Autodesk Inventor part; units mm, degrees
ref_plane "YZ Plane" through (0, 0, 0) normal (1, 0, 0) x (0, 1, 0)
ref_plane "XZ Plane" through (0, 0, 0) normal (0, 1, 0) x (-1, 0, 0)
ref_plane "XY Plane" through (0, 0, 0) normal (0, 0, 1) x (1, 0, 0)
sketch "草图1" plane through (0, 0, 0) normal (0, 1, 0) x (-1, 0, 0)
  circle A0 centre (0, 0) radius 1.5
  line L0 (0, 0) -> (-13.1253, 0) construction
  circle A1 centre (-4.1, 0) radius 0.5
  circle A2 centre (-6.2, 0) radius 0.5
  circle A3 centre (-8.3, 0) radius 0.5
  circle A4 centre (-10.4, 0) radius 0.5
  circle A5 centre (-12.5, 0) radius 0.5
  circle A6 centre (-14.6, 0) radius 0.5
  arc A7 (-0.4195, -3.4748) -> (-0.4195, 3.4748) centre (0, 0) ccw
  arc A8 (-14.8098, 1.7374) -> (-14.8098, -1.7374) centre (-14.6, 0) ccw
  line L1 (-0.4195, -3.4748) -> (-14.8098, -1.7374)
  line L2 (-0.4195, 3.4748) -> (-14.8098, 1.7374)
  dimension "d0" = 3
  dimension "d1" = 1
  dimension "d2" = 4.1
  dimension "d5" = 2.1
  dimension "d10" = 7
  dimension "d11" = 3.5
extrude "拉伸1" add sketch "草图1" along normal blind 1.5
sketch "草图2" plane through (0, 1.5, 0) normal (0, 1, 0) x (1, 0, 0)
  circle A0 centre (0, 0) radius 3.5
  line L0 (0.4195, -3.4748) -> (14.8098, -1.7374)
  arc A1 (14.8098, -1.7374) -> (14.8098, 1.7374) centre (14.6, 0) ccw
  line L1 (14.8098, 1.7374) -> (0.4195, 3.4748)
  arc A2 (0.4195, 3.4748) -> (0.4195, -3.4748) centre (0, 0) ccw
  circle A3 centre (4.1, 0) radius 0.5
  circle A4 centre (6.2, 0) radius 0.5
  circle A5 centre (8.3, 0) radius 0.5
  circle A6 centre (10.4, 0) radius 0.5
  circle A7 centre (12.5, 0) radius 0.5
  circle A8 centre (14.6, 0) radius 0.5
  circle A9 centre (0, 0) radius 1.5
  circle A10 centre (0, 0) radius 2.5
  dimension "d16" = 5
extrude "拉伸2" add sketch "草图2" along normal blind 2.5 contours A0
properties part number "sg90舵盘01"
Read the model definition and answer for the solid it produces. Units are mm, in the model's axes. A direction names the side the tool comes from. Coordinates: 2 decimals unless noted, no trailing zeros. Write each loop counter-clockwise with the first axis right and the second up, starting at its lowest first coordinate (ties: lowest second). Pieces come first, ordered by that corner, then holes. Notation, with made-up numbers: (-12.75, -8.75) - (-7.75, -8.75) arc R22 ccw to (-7.75, 2.25) - close; hole circle Ø2 at (83.5, -20.5). An arc over 180 degrees is marked (long way). Answer as a JSON object with one key per item and string values. Group by question number.
1. This flat-tipped pin is pushed along its axis until it touches: P1, Ø2, axis at x = 0, z = -1, coming from the +Y side. Where does it stop, or does it pass through?
2. Which of the six approach directions +Z, -Z, +X, -X, +Y, -Y give full straight-line access (tool end or side, diameter ignored) to faces 1 (the cylindrical face through (3.233, 2.732, -1.341)), 2 (the cylindrical face through (1.5, 0.74, -0.07))?
3. The mould has two halves that part along X. Classify faces 3 (the cylindrical face through (10.9, 0.7, 0)), 4 (the cylindrical face through (16.35, 0.74, -0.04)), 5 (the flat face through (-2, 1.5, 0)), 6 (the flat face through (2, 4, 2)): +X half, -X half, draft (parallel to the pull), parting line (faces both ways), or undercut.
4. A cutting plane is placed at C-C (z = 1). Determine the outline of the cut face in (x, y), plus the area to 3 significant figures.
5. A cutting plane is placed at A-A (x = 0). Determine the outline of the cut face in (y, z).
6. A cutting plane is placed at D-D (z = 0). Give the number of separate pieces and of enclosed holes in the cut face, plus the area to 3 significant figures.
7. Consider L1, parallel to Z at x = 0, y = 2.6; L2, parallel to Y at x = 6.5, z = -0.75. Determine where each line is inside the solid, lowest interval first. Write a range as [from, to].
8. A cutting plane is placed at B-B (y = 0.55). Determine the outline of the cut face in (x, z), plus the area to 3 significant figures.
Worked out:
{
 "1": {"P1": "stops at y = 1.5"},
 "2": {"face 1": "+Y", "face 2": "+Y, -Y"},
 "3": {"face 3": "undercut", "face 4": "+X half", "face 5": "undercut", "face 6": "draft"},
 "4": {"outline": "(-3.35, 0) - (-1.12, 0) - (-1.12, 1.5) - (-2.29, 1.5) - (-2.29, 4) - (-3.35, 4) - close; (1.12, 0) - (16.04, 0) - (16.04, 1.5) - (3.35, 1.5) - (3.35, 4) - (2.29, 4) - (2.29, 1.5) - (1.12, 1.5) - close", "area": "31.0 mm²"},
 "5": {"outline": "(0, -3.5) - (4, -3.5) - (4, -2.5) - (1.5, -2.5) - (1.5, -1.5) - (0, -1.5) - close; (0, 1.5) - (1.5, 1.5) - (1.5, 2.5) - (4, 2.5) - (4, 3.5) - (0, 3.5) - close"},
 "6": {"separate pieces": "8", "enclosed holes": "0", "area": "21.3 mm²"},
 "7": {"L1": "z = [-3.5, -2.5], [2.5, 3.5]", "L2": "y = [0, 1.5]"},
 "8": {"outline": "(0.42, -3.47) - (14.81, -1.74) arc R1.75 ccw to (14.81, 1.74) - (0.42, 3.47) arc R3.5 ccw (long way) to start; hole circle Ø3 at (0, 0); hole circle Ø1 at (4.1, 0); hole circle Ø1 at (6.2, 0); hole circle Ø1 at (8.3, 0); hole circle Ø1 at (10.4, 0); hole circle Ø1 at (12.5, 0); hole circle Ø1 at (14.6, 0)", "area": "89.5 mm²"}
}
